from build123d import *

# Parameters (mm, degrees)
F0_R        = 5.5
F0_R_2      = 21.2
F1_DEPTH    = 6
F2_T1_DEPTH = 47.7037001686
F2_T3_DEPTH = 29.5051884552


# Not quite as in the source:
# - a fillet or chamfer that OpenCascade refuses, or shapes differently, is made with other operations: its cross-section is extruded or revolved along the edge and cut away or added


with BuildPart() as f1:
    # F0 (on Top) → F1 (new body, symmetric)
    with BuildSketch(Plane.XY):
        Polygon((103.0366095362, 47.75), (-103.0366095362, 47.75), (-132.5, -33.2), (0, -33.2), (132.5, -33.2), align=None)
        with Locations((-117.5, -25.7)):
            Circle(F0_R, mode=Mode.SUBTRACT)
        with Locations((-58.5, -25.7)):
            Circle(F0_R, mode=Mode.SUBTRACT)
        with Locations((-29.5, -25.7)):
            Circle(F0_R, mode=Mode.SUBTRACT)
        with Locations((-88, 0)):
            Circle(F0_R_2, mode=Mode.SUBTRACT)
        with Locations((29.5, -25.7)):
            Circle(F0_R, mode=Mode.SUBTRACT)
        with Locations((58.5, -25.7)):
            Circle(F0_R, mode=Mode.SUBTRACT)
        with Locations((117.5, -25.7)):
            Circle(F0_R, mode=Mode.SUBTRACT)
        Circle(F0_R_2, mode=Mode.SUBTRACT)
        with Locations((88, 0)):
            Circle(F0_R_2, mode=Mode.SUBTRACT)
        with Locations((-88, 36.25)):
            Circle(F0_R, mode=Mode.SUBTRACT)
        with Locations((0, 36.25)):
            Circle(F0_R, mode=Mode.SUBTRACT)
        with Locations((88, 36.25)):
            Circle(F0_R, mode=Mode.SUBTRACT)
    extrude(amount=F1_DEPTH, both=True)

    # F2: fillet of radius 5 on 4 edges, made by hand

    # F2_s2 → F2_t1 (cut)
    with BuildSketch(Plane.XY.offset(-23.8518500843)):
        with BuildLine():
            add(Edge.make_bspline(
                [(-125.3592599663, -33.2), (-132.5, -33.2), (-130.0577230702, -26.4898992834)],
                knots=[0, 0, 0, 1, 1, 1], degree=2, weights=[1, 1, 1]))
            Line((-130.0577230702, -26.4898992834), (-132.5, -33.2))
            Line((-132.5, -33.2), (-125.3592599663, -33.2))
        make_face()
        with BuildLine():
            add(Edge.make_bspline(
                [(130.0577230702, -26.4898992834), (132.5, -33.2), (125.3592599663, -33.2)],
                knots=[0, 0, 0, 1, 1, 1], degree=2, weights=[1, 1, 1]))
            Line((125.3592599663, -33.2), (132.5, -33.2))
            Line((132.5, -33.2), (130.0577230702, -26.4898992834))
        make_face()
    extrude(amount=F2_T1_DEPTH, mode=Mode.SUBTRACT)

    # F2_s4 → F2_t3 (cut)
    with BuildSketch(Plane.XY.offset(-14.7525942276)):
        with BuildLine():
            add(Edge.make_bspline(
                [(-99.5355718451, 47.75), (-103.0366095362, 47.75), (-104.234034949, 44.4601007166)],
                knots=[0, 0, 0, 1, 1, 1], degree=2, weights=[1, 1, 1]))
            Line((-104.234034949, 44.4601007166), (-103.0366095362, 47.75))
            Line((-103.0366095362, 47.75), (-99.5355718451, 47.75))
        make_face()
        with BuildLine():
            add(Edge.make_bspline(
                [(99.5355718451, 47.75), (103.0366095362, 47.75), (104.234034949, 44.4601007166)],
                knots=[0, 0, 0, 1, 1, 1], degree=2, weights=[1, 1, 1]))
            Line((104.234034949, 44.4601007166), (103.0366095362, 47.75))
            Line((103.0366095362, 47.75), (99.5355718451, 47.75))
        make_face()
    extrude(amount=F2_T3_DEPTH, mode=Mode.SUBTRACT)


solid = f1.part
The listing builds one solid part. Answer for the finished solid, in the listing's coordinates (mm). Coordinates: 2 decimals unless noted, no trailing zeros. Write each loop counter-clockwise with the first axis right and the second up, starting at its lowest first coordinate (ties: lowest second). Pieces come first, ordered by that corner, then holes. Notation, with made-up numbers: (60, 46) -> (70, 46) arc R24 cw to (70, 74) -> close; hole circle Ø7 at (11.25, 46.25). An arc over 180 degrees is marked (long way). One line per question, with ' | ' between items.
1. For a pull along X with two mould halves and no side action, classify faces 1 (the flat face through (117.327, 8.488, 0.084)), 2 (the flat face through (1, 47.75, 0)), 3 (the cylindrical face through (-93.495, 36.492, -0.084)), 4 (the flat face through (-116.965, 9.482, 0.084)) as released by +X, released by -X, zero draft, split by the parting line, or undercut.
Verdict:
face 1: released by +X | face 2: zero draft | face 3: undercut | face 4: released by -X
2. Section C-C (x = 117.5) is taken. Determine the outline of the cut face in (y, z), and give its area (3 significant figures).
Verdict:
outline: (-33.2, -6) -> (-31.2, -6) -> (-31.2, 6) -> (-33.2, 6) -> close; (-20.2, -6) -> (8.01, -6) -> (8.01, 6) -> (-20.2, 6) -> close | area: 363 mm^2
3. Given pin 1 Ø1.5 at (y, z) = (34, 0.5) entering from +X; pin 2 Ø9 at (x, y) = (-88, 36.25) entering from -Z; pin 3 Ø4 at (y, z) = (33.5, -2.5) entering from -X; pin 4 Ø2 at (y, z) = (-13, 0) entering from -X, each flat-ended and moving along its own axis, determine where each tip first touches the part or whether it passes through.
Verdict:
pin 1: stops at x = 108.31 | pin 2: passes through | pin 3: stops at x = -108.95 | pin 4: stops at x = -125.51
4. Section D-D (z = 0.25) is taken. State how many separate pieces and enclosed holes the cut face has, and give its area (3 significant figures).
Verdict:
separate pieces: 1 | enclosed holes: 12 | area: 14,000 mm^2
5. Section B-B (y = 34) is taken. Determine the outline of the cut face in (x, z).
Verdict:
outline: (-108.04, -6) -> (-93.02, -6) -> (-93.02, 6) -> (-108.04, 6) -> close; (-82.98, -6) -> (-5.02, -6) -> (-5.02, 6) -> (-82.98, 6) -> close; (5.02, -6) -> (82.98, -6) -> (82.98, 6) -> (5.02, 6) -> close; (93.02, -6) -> (108.04, -6) -> (108.04, 6) -> (93.02, 6) -> close
6. Section A-A (x = -88) is taken. Determine the outline of the cut face in (y, z).
Verdict:
outline: (-33.2, -6) -> (-21.2, -6) -> (-21.2, 6) -> (-33.2, 6) -> close; (21.2, -6) -> (30.75, -6) -> (30.75, 6) -> (21.2, 6) -> close; (41.75, -6) -> (47.75, -6) -> (47.75, 6) -> (41.75, 6) -> close
7. Straight lines are drawn through the part: line 1 (Y direction, x = -88, z = 0.25); line 2 (Y direction, x = 2.5, z = -0.5); line 3 (X direction, y = -13.5, z = 2). For each, find the intervals that lie inside material, in ascending order.
Verdict:
line 1: y = -33.2 to -21.2, 21.2 to 30.75, 41.75 to 47.75 | line 2: y = -33.2 to -21.05, 21.05 to 31.35, 41.15 to 47.75 | line 3: x = -125.33 to -104.35, -71.65 to -16.35, 16.35 to 71.65, 104.35 to 125.33
